Source: CAD feature listing. Evaluate the final solid. Frame: model axes, mm. Coordinates: 2 decimals unless noted, no trailing zeros. Loops run counter-clockwise (first coordinate to the right, second up) from the corner with the lowest first, then second, coordinate; pieces in that order, holes last. Notation, with made-up numbers: M 3.25,-6 L 43.25,-6 A25 cw 43.25,32 Z; hole C 53,-17 d1. An arc over 180 degrees is marked long. One line per question, with ' | ' between items. Start each with the question number.
1. Pin query (flat end, axial travel): P1, Ø1, axis at x = 9, y = 4.5, coming from the +Z side; P2, Ø1, axis at y = 5.5, z = 35, coming from the +X side (3 decimals); P3, Ø4, axis at x = 3, z = 148.5, coming from the +Y side. Return the tip coordinate at first contact, or that it passes through.
2. Mould query, pull axis X, two halves, no side actions, for faces 1 (the flat face through (0, 0, 101)), 2 (the cylindrical face through (0, 8, 106)). Classes: pulls with the +X half, pulls with the -X half, needs draft (parallel to the pull), parting line crosses it, or undercut.
3. Ray query, probe 1 along Y at (x, z) = (0, 116); probe 2 along Y at (x, z) = (-4.5, 125); probe 3 along X at (y, z) = (1, 61). Return the intervals inside material, ascending.
4. Section query A-A, the plane z = 57. Output: boundary loops of the cut face in (x, y), and give its area (3 significant figures).
```python
from build123d import *

# Parameters (mm, degrees)
F1_DEPTH    = 5
F2_DEPTH    = 200
F3_T2_ANGLE = 180
F4_T2_ANGLE = 275.6465366004


# Not quite as in the source:
# - a fillet or chamfer that OpenCascade refuses, or shapes differently, is made with other operations: its cross-section is extruded or revolved along the edge and cut away or added


with BuildPart() as f1:
    # F0 (on Top) → F1 (new body)
    with BuildSketch(Plane.XY):
        with BuildLine():
            ThreePointArc((15, 0), (0, 15), (-15, 0))
            Line((-15, 0), (-8, 0))
            ThreePointArc((-8, 0), (0, 8), (8, 0))
            Line((8, 0), (15, 0))
        make_face()
        with BuildLine():
            ThreePointArc((8, 0), (0, 8), (-8, 0))
            Line((-8, 0), (8, 0))
        make_face()
    extrude(amount=F1_DEPTH)

    # F0 (on Top) → F2 (join)
    with BuildSketch(Plane.XY):
        with BuildLine():
            ThreePointArc((8, 0), (0, 8), (-8, 0))
            Line((-8, 0), (8, 0))
        make_face()
    extrude(amount=F2_DEPTH)

    # F3: fillet of radius 10 on 1 edges, made by hand

    # F3_s1 → F3_t2 (revolve)
    with BuildSketch(Plane.XZ):
        with BuildLine():
            ThreePointArc((-8, 14.5393920142), (-9.9377422517, 8.6233122311), (-15, 5))
            Line((-15, 5), (-8, 5))
            Line((-8, 5), (-8, 14.5393920142))
        make_face()
    revolve(axis=Axis((0, 0, 5), (0, 0, -1)), revolution_arc=F3_T2_ANGLE)

    # F4: fillet of radius 10 on 1 edges, made by hand

    # F4_s1 → F4_t2 (revolve, cut)
    with BuildSketch(Plane(origin=(0, 0, 0), x_dir=(0, 0, 1), z_dir=(-0.7410773266, -0.6714196869, 0))):
        with BuildLine():
            ThreePointArc((0, -15), (3.8172075141, -13.9552733931), (6.9301950027, -11.511539409))
            ThreePointArc((6.9301950027, -11.511539409), (5.7894854023, -13.1586020321), (5, -15))
            Line((5, -15), (0, -15))
        make_face()
    revolve(axis=Axis((0, 0, 5), (0, 0, 1)), revolution_arc=F4_T2_ANGLE, mode=Mode.SUBTRACT)


solid = f1.part
```
Taken from the geometry:
1) P1: z = 9.17 | P2: x = 6.245 | P3: y = 7.94
2) face 1: needs draft | face 2: parting line crosses it
3) probe 1: 0 to 8 | probe 2: 0 to 6.61 | probe 3: -7.94 to 7.94
4) outline: M -8,0 L 8,0 A8 ccw Z | area: 101 mm^2
